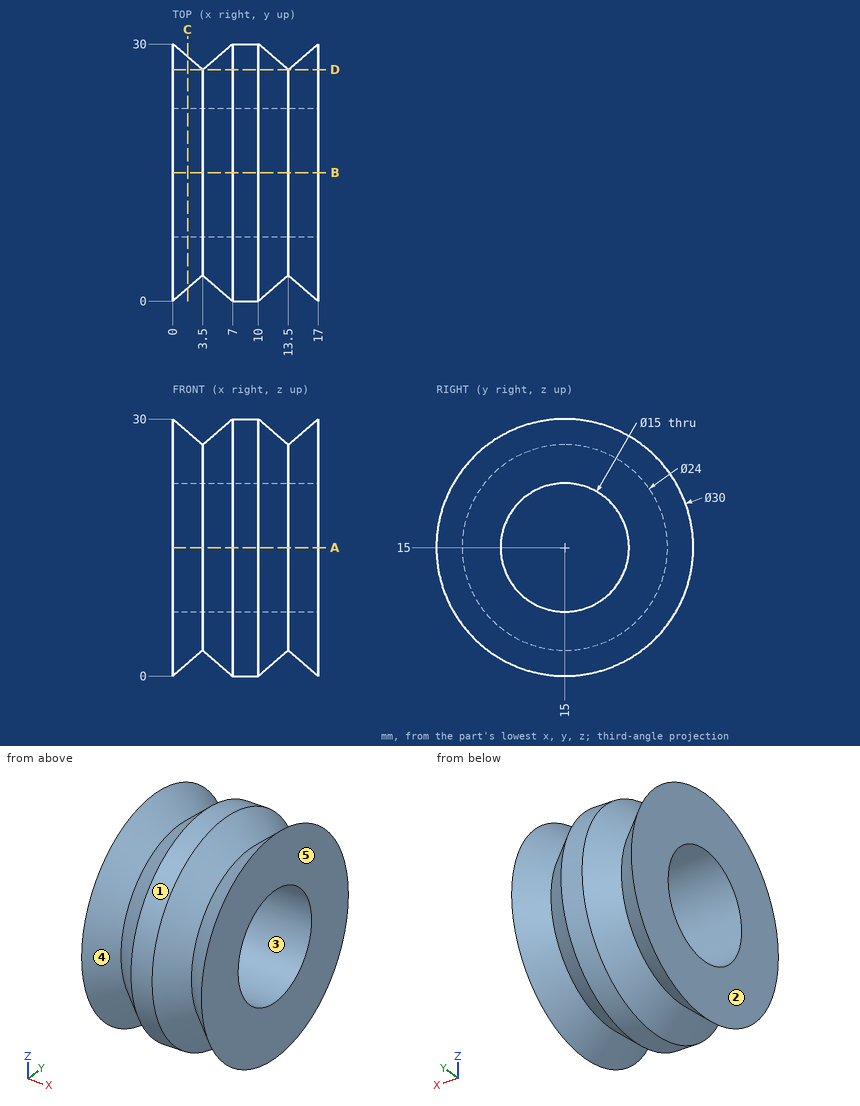
Job drawing, mm, ordinate dimensions from the low corner. One solid piece. A direction names the side the tool comes from. Coordinates: 2 decimals unless noted, no trailing zeros. Write each loop counter-clockwise with the first axis right and the second up, starting at its lowest first coordinate (ties: lowest second). Pieces come first, ordered by that corner, then holes. Notation, with made-up numbers: (34.5, 47) - (54.5, 47) arc R24 cw to (54.5, 75) - close; hole circle Ø5 at (21.5, 74.25). An arc over 180 degrees is marked (long way). Use a Markdown table: item, result. Add a question column.
Item 1: Band-saw the part on C-C, the plane x = 1.75. Give the cut face in (y, z), and give its area (3 significant figures).
Item 2: Flat gauge pins, fed straight in: pin 1 (1 mm diameter, centred on x = 9, y = 3.5, fed in from -Z); pin 2 (4 mm diameter, centred on x = 11.5, z = 9.5, fed in from +Y); pin 3 (5 mm diameter, centred on x = 6.5, y = 12, fed in from +Z). Where does each tip first touch, or does it go through?
Item 3: Band-saw the part on A-A, the plane z = 15. Give the cut face in (x, y).
Item 4: Band-saw the part on D-D, the plane y = 27. Give the number of separate pieces and of enclosed holes in the cut face, and give its area (3 significant figures).
Item 5: Drill centre lines: L1, parallel to X at y = 11.5, z = 27.5; L2, parallel to Y at x = 8, z = 15; L3, parallel to X at y = 13.25, z = 3. Where is each one in solid material? Low to high. Write a range as from..to.
Item 6: Mould opens along Y. For the marked faces 1, 2 and 3 say: pulls with the +Y half, pulls with the -Y half, needs draft (parallel to the pull), parting line crosses it, or undercut.
Item 7: 3-axis set-ups, long thin cutter, end or side, ignore diameter. For the marked faces 4 and 5: which of +Z, -Z, +X, -X, +Y, -Y reach the whole face in a straight line?
Numbers:
| question | item | result |
|---|---|---|
| 1 | outline | circle Ø27 at (15, 15); hole circle Ø15 at (15, 15) |
| 1 | area | 396 mm2 |
| 2 | pin 1 | z = 4.8 |
| 2 | pin 2 | y = 29.41 |
| 2 | pin 3 | z = 29.99 |
| 3 | outline | (0, 0) - (3.5, 3) - (7, 0) - (10, 0) - (13.5, 3) - (17, 0) - (17, 7.5) - (0, 7.5) - close; (0, 22.5) - (17, 22.5) - (17, 30) - (13.5, 27) - (10, 30) - (7, 30) - (3.5, 27) - (0, 30) - close |
| 4 | separate pieces | 3 |
| 4 | enclosed holes | 0 |
| 4 | area | 218 mm2 |
| 5 | L1 | 0..2.36, 4.64..12.36, 14.64..17 |
| 5 | L2 | 0..7.5, 22.5..30 |
| 5 | L3 | 0..3.35, 3.65..13.35, 13.65..17 |
| 6 | face 1 | parting line crosses it |
| 6 | face 2 | needs draft |
| 6 | face 3 | undercut |
| 7 | face 4 | none |
| 7 | face 5 | +Z, -Z, +X, +Y, -Y |
